Geometry check sheet. Reference: the model listing, model coordinates, mm. A direction names the side the tool comes from. Round coordinates to 2 decimals unless told otherwise and drop trailing zeros. Loops run counter-clockwise (first coordinate to the right, second up) from the corner with the lowest first, then second, coordinate; pieces in that order, holes last. Notation, with made-up numbers: M 83.5,-18 L 133.5,-18 A33 cw 133.5,16 Z; hole C 47,78.5 d3. An arc over 180 degrees is marked long. Use one line per item in the form item = value. Start each with the question number.
1. Cross-section at D-D (z = 38.5). Record the boundary of the cut face in (x, y).
2. Draft check along Z on faces 6 (the flat face through (-6, -660.4, 1)), 7 (the flat face through (-27.134, -325.577, -25.664)), 8 (the flat face through (-42, -326, 10.99)). Enter one of: pulls with the +Z half, pulls with the -Z half, needs draft (parallel to the pull), parting line crosses it, or undercut.
3. Cross-section at C-C (x = -43.5). Record the boundary of the cut face in (y, z), then the cut area to 3 significant figures.
4. Cross-section at A-A (z = -31.5). Record the boundary of the cut face in (x, y).
5. Set-up check for faces 1 (the flat face through (16.17, -325.58, 19.59)), 2 (the flat face through (5.789, -325.577, -36.652)), 3 (the flat face through (-6, 0, 1)), 4 (the flat face through (-16.484, -326, 30)), 5 (the flat face through (30, -326, -9.158)): record each of +Z, -Z, +X, -X, +Y, -Y from which the full face is reachable in a straight line by a thin tool's end or side.
6. Cross-section at B-B (y = -547). Record the boundary of the cut face in (x, z).
7. Go/stop test with flat-tipped pins: pin 1 (5 mm diameter, centred on x = 25, y = -273.5, fed in from -Z); pin 2 (4 mm diameter, centred on x = 36, y = -209, fed in from +Z); pin 3 (6 mm diameter, centred on x = -35.5, y = -310.5, fed in from -Z). Record where each tip stops, or that it passes through.
8. Material ranges on line 1 (X direction, y = -429.5, z = -42); line 2 (X direction, y = -598.5, z = -29); line 3 (Z direction, x = 30, y = -347), recorded low to high.
```python
from build123d import *

# Parameters (mm, degrees)
F1_DEPTH = 25.4
F2_DEPTH = 609.6
F3_DEPTH = 25.4


with BuildPart() as f1:
    # F0 (on Front) → F1 (new body)
    with BuildSketch(Plane.XZ):
        Polygon((-28.0406700106, -48.6028654858), (-7.6316785999, -25.0319186598), (19.5911039028, -48.6028654858), (13.1264980882, -9.1580180451), (47.9269810021, -9.1580180451), (-16.4844300598, 49.1480454803), (-16.4844300598, 10.9896259382), (-68.3798789978, 10.9896259382), (-26.2529868633, -3.3579384908), align=None)
    extrude(amount=F1_DEPTH)

    # F2 (add): a face of the model
    f2_faces = [f1.faces().sort_by_distance(p)[0] for p in [
        (-3.7729101516, -25.4, -1.8402904119),
    ]]
    extrude(f2_faces, amount=F2_DEPTH)

    # F3 (add): a face of the model
    f3_faces = [f1.faces().sort_by_distance(p)[0] for p in [
        (-3.7729101516, -635, -1.8402904119),
    ]]
    extrude(f3_faces, amount=F3_DEPTH)


solid = f1.part
```
Reported:
q1.outline = M -16.48,-660.4 L -4.72,-660.4 L -4.72,0 L -16.48,0 Z
q2.face_6 = needs draft
q2.face_7 = undercut
q2.face_8 = pulls with the +Z half
q3.outline = M -660.4,2.52 L 0,2.52 L 0,10.99 L -660.4,10.99 Z
q3.area = 5,600 mm²
q4.outline = M -27.36,-660.4 L -13.23,-660.4 L -13.23,0 L -27.36,0 Z; M -0.16,-660.4 L 16.79,-660.4 L 16.79,0 L -0.16,0 Z
q5.face_1 = +Z, +X, +Y, -Y
q5.face_2 = -Z, +Y, -Y
q5.face_3 = +Z, -Z, +X, -X, +Y
q5.face_4 = +Z, -X, +Y, -Y
q5.face_5 = +X, +Y, -Y
q6.outline = M -68.38,10.99 L -26.25,-3.36 L -28.04,-48.6 L -7.63,-25.03 L 19.59,-48.6 L 13.13,-9.16 L 47.93,-9.16 L -16.48,49.15 L -16.48,10.99 Z
q7.pin_1 = -9.16
q7.pin_2 = 3.45
q7.pin_3 = -1.23
q8.line_1 = -27.78 to -22.32, 11.97 to 18.51
q8.line_2 = -27.27 to -11.07, -3.05 to 16.38
q8.line_3 = -9.16 to 7.07
